Could you check a few things on this model? Use its own coordinates, in mm. A direction names the side the tool comes from. Round coordinates to 2 decimals unless told otherwise and drop trailing zeros. Order: outer loops, then holes, each group sorted by start corner. A loop starts at its lowest first (then second) coordinate and runs counter-clockwise, first axis right, second up. Notation, with made-up numbers: (37.25, -2) -> (45.25, -2) arc R9 cw to (45.25, 5) -> close; hole circle Ø2 at (72.5, -20). An arc over 180 degrees is marked (long way). One line per question, with ' | ' between items.
```python
from build123d import *

# Parameters (mm, degrees)
CYLINDER025_R          = 1
CYLINDER025_DEPTH      = 96
CYLINDER025_ROLL_ANGLE = -33
CYLINDER020_R          = 2
CYLINDER020_DEPTH      = 16
CYLINDER024_R          = 3
CYLINDER024_DEPTH      = 16
CYLINDER022_R          = 3
CYLINDER022_DEPTH      = 16
BOX021_W               = 26
BOX021_H               = 23
BOX021_DEPTH           = 13
CYLINDER011_R          = 1.9
CYLINDER011_DEPTH      = 12
CYLINDER012_R          = 1.9
CYLINDER012_DEPTH      = 12
CYLINDER013_R          = 1.9
CYLINDER013_DEPTH      = 12
CYLINDER014_R          = 1.9
CYLINDER014_DEPTH      = 12
BOX008_W               = 41
BOX008_H               = 20
BOX008_DEPTH           = 12
BOX019_W               = 10
BOX019_H               = 10
BOX019_DEPTH           = 10
BOX019_PLACEMENT_ANGLE = 8
BOX018_W               = 14
BOX018_H               = 10
BOX018_DEPTH           = 10
BOX018_PLACEMENT_ANGLE = 16
BOX017_W               = 65
BOX017_H               = 11
BOX017_DEPTH           = 10
BOX017_PLACEMENT_ANGLE = 15
BOX016_W               = 76
BOX016_H               = 10
BOX016_DEPTH           = 10
BOX015_W               = 49
BOX015_H               = 10
BOX015_DEPTH           = 10
BOX015_PLACEMENT_ANGLE = -19
BOX014_W               = 53
BOX014_H               = 10
BOX014_DEPTH           = 10
BOX014_PLACEMENT_ANGLE = -36
BOX013_W               = 13
BOX013_H               = 11
BOX013_DEPTH           = 10
BOX012_W               = 23
BOX012_H               = 17
BOX012_DEPTH           = 10
BOX011_W               = 41
BOX011_H               = 6
BOX011_DEPTH           = 10
CYLINDER016_R          = 43
CYLINDER016_DEPTH      = 10
CYLINDER015_R          = 13
CYLINDER015_DEPTH      = 10
BOX010_W               = 37
BOX010_H               = 8
BOX010_DEPTH           = 12
BOX009_W               = 184
BOX009_H               = 34
BOX009_DEPTH           = 6
CHAMFER_SIZE           = 6
CHAMFER001_SIZE        = 1
CUT025_PITCH_ANGLE     = 90
FILLET_R               = 3
FILLET001_R            = 3
CUT035_ROLL_ANGLE      = -45
BOX024_W               = 10
BOX024_H               = 10
BOX024_DEPTH           = 13
CHAMFER002_SIZE        = 3
CHAMFER003_SIZE        = 3


with BuildPart() as cylinder025:
    # Cylinder025 → Cylinder025 (new body)
    with BuildSketch(Plane.XY):
        Circle(CYLINDER025_R)
    extrude(amount=CYLINDER025_DEPTH)


with BuildPart() as cylinder025_1:
    # Cylinder025 roll: moved
    add(cylinder025.part.rotate(Axis((0, 0, 0), (1, 0, 0)), CYLINDER025_ROLL_ANGLE))


with BuildPart() as cylinder025_2:
    # Cylinder025 placement: moved
    add(cylinder025_1.part.moved(Location((-2.5, 14, 31))))


with BuildPart() as cylinder020:
    # Cylinder020 → Cylinder020 (new body)
    with BuildSketch(Plane.XY.offset(9)):
        Circle(CYLINDER020_R)
    extrude(amount=CYLINDER020_DEPTH)


with BuildPart() as cylinder024:
    # Cylinder024 → Cylinder024 (new body)
    with BuildSketch(Plane.XY.offset(23)):
        Circle(CYLINDER024_R)
    extrude(amount=CYLINDER024_DEPTH)


with BuildPart() as not_used_cylinder001:
    # Cylinder022 → Cylinder022 (new body)
    with BuildSketch(Plane(origin=(0, -50, 23), x_dir=(1, 0, 0), z_dir=(0, 0, 1))):
        Circle(CYLINDER022_R)
    extrude(amount=CYLINDER022_DEPTH)


with BuildPart() as cube021:
    # Box021 → Box021 (new body)
    with BuildSketch(Plane(origin=(161, 15, -3), x_dir=(1, 0, 0), z_dir=(0, 0, 1))):
        with Locations((13, 11.5)):
            Rectangle(BOX021_W, BOX021_H)
    extrude(amount=BOX021_DEPTH)


with BuildPart() as cylinder011:
    # Cylinder011 → Cylinder011 (new body)
    with BuildSketch(Plane(origin=(38, 19.5, -1), x_dir=(1, 0, 0), z_dir=(0, 0, 1))):
        Circle(CYLINDER011_R)
    extrude(amount=CYLINDER011_DEPTH)


with BuildPart() as cylinder012:
    # Cylinder012 → Cylinder012 (new body)
    with BuildSketch(Plane(origin=(38, 29, -1), x_dir=(1, 0, 0), z_dir=(0, 0, 1))):
        Circle(CYLINDER012_R)
    extrude(amount=CYLINDER012_DEPTH)


with BuildPart() as cylinder013:
    # Cylinder013 → Cylinder013 (new body)
    with BuildSketch(Plane(origin=(87, 29, -1), x_dir=(1, 0, 0), z_dir=(0, 0, 1))):
        Circle(CYLINDER013_R)
    extrude(amount=CYLINDER013_DEPTH)


with BuildPart() as cylinder014:
    # Cylinder014 → Cylinder014 (new body)
    with BuildSketch(Plane(origin=(87, 19.5, -1), x_dir=(1, 0, 0), z_dir=(0, 0, 1))):
        Circle(CYLINDER014_R)
    extrude(amount=CYLINDER014_DEPTH)


with BuildPart() as cube008:
    # Box008 → Box008 (new body)
    with BuildSketch(Plane(origin=(42, 14, -1), x_dir=(1, 0, 0), z_dir=(0, 0, 1))):
        with Locations((20.5, 10)):
            Rectangle(BOX008_W, BOX008_H)
    extrude(amount=BOX008_DEPTH)


with BuildPart() as cube019:
    # Box019 → Box019 (new body)
    with BuildSketch(Plane.XY):
        with Locations((5, 5)):
            Rectangle(BOX019_W, BOX019_H)
    extrude(amount=BOX019_DEPTH)


with BuildPart() as cube019_1:
    # Box019 placement: moved
    add(cube019.part.moved(Location((106, -7, 0))).rotate(Axis((106, -7, 0), (0, 0, 1)), BOX019_PLACEMENT_ANGLE))


with BuildPart() as cube018:
    # Box018 → Box018 (new body)
    with BuildSketch(Plane.XY):
        with Locations((7, 5)):
            Rectangle(BOX018_W, BOX018_H)
    extrude(amount=BOX018_DEPTH)


with BuildPart() as cube018_1:
    # Box018 placement: moved
    add(cube018.part.moved(Location((174, 10, 0))).rotate(Axis((174, 10, 0), (0, 0, 1)), BOX018_PLACEMENT_ANGLE))


with BuildPart() as cube017:
    # Box017 → Box017 (new body)
    with BuildSketch(Plane.XY):
        with Locations((32.5, 5.5)):
            Rectangle(BOX017_W, BOX017_H)
    extrude(amount=BOX017_DEPTH)


with BuildPart() as cube017_1:
    # Box017 placement: moved
    add(cube017.part.moved(Location((115, -7, 0))).rotate(Axis((115, -7, 0), (0, 0, 1)), BOX017_PLACEMENT_ANGLE))


with BuildPart() as cube016:
    # Box016 → Box016 (new body)
    with BuildSketch(Plane(origin=(46, -7, 0), x_dir=(1, 0, 0), z_dir=(0, 0, 1))):
        with Locations((38, 5)):
            Rectangle(BOX016_W, BOX016_H)
    extrude(amount=BOX016_DEPTH)


with BuildPart() as cube015:
    # Box015 → Box015 (new body)
    with BuildSketch(Plane.XY):
        with Locations((24.5, 5)):
            Rectangle(BOX015_W, BOX015_H)
    extrude(amount=BOX015_DEPTH)


with BuildPart() as cube015_1:
    # Box015 placement: moved
    add(cube015.part.moved(Location((16, 5, 0))).rotate(Axis((16, 5, 0), (0, 0, 1)), BOX015_PLACEMENT_ANGLE))


with BuildPart() as cube014:
    # Box014 → Box014 (new body)
    with BuildSketch(Plane.XY):
        with Locations((26.5, 5)):
            Rectangle(BOX014_W, BOX014_H)
    extrude(amount=BOX014_DEPTH)


with BuildPart() as cube014_1:
    # Box014 placement: moved
    add(cube014.part.moved(Location((-16, 28, 0))).rotate(Axis((-16, 28, 0), (0, 0, 1)), BOX014_PLACEMENT_ANGLE))


with BuildPart() as cube013:
    # Box013 → Box013 (new body)
    with BuildSketch(Plane(origin=(0, 8, 0), x_dir=(1, 0, 0), z_dir=(0, 0, 1))):
        with Locations((6.5, 5.5)):
            Rectangle(BOX013_W, BOX013_H)
    extrude(amount=BOX013_DEPTH)


with BuildPart() as cube012:
    # Box012 → Box012 (new body)
    with BuildSketch(Plane(origin=(161, 0, 0), x_dir=(1, 0, 0), z_dir=(0, 0, 1))):
        with Locations((11.5, 8.5)):
            Rectangle(BOX012_W, BOX012_H)
    extrude(amount=BOX012_DEPTH)


with BuildPart() as cube011:
    # Box011 → Box011 (new body)
    with BuildSketch(Plane(origin=(120, 0, 0), x_dir=(1, 0, 0), z_dir=(0, 0, 1))):
        with Locations((20.5, 3)):
            Rectangle(BOX011_W, BOX011_H)
    extrude(amount=BOX011_DEPTH)


with BuildPart() as cylinder016:
    # Cylinder016 → Cylinder016 (new body)
    with BuildSketch(Plane(origin=(132, 63, 0), x_dir=(1, 0, 0), z_dir=(0, 0, 1))):
        Circle(CYLINDER016_R)
    extrude(amount=CYLINDER016_DEPTH)


with BuildPart() as cylinder015:
    # Cylinder015 → Cylinder015 (new body)
    with BuildSketch(Plane(origin=(20, 37, 0), x_dir=(1, 0, 0), z_dir=(0, 0, 1))):
        Circle(CYLINDER015_R)
    extrude(amount=CYLINDER015_DEPTH)


with BuildPart() as cube010:
    # Box010 → Box010 (new body)
    with BuildSketch(Plane.XY):
        with Locations((18.5, 4)):
            Rectangle(BOX010_W, BOX010_H)
    extrude(amount=BOX010_DEPTH)


with BuildPart() as cut035:
    # Box009 → Box009 (new body)
    with BuildSketch(Plane.XY):
        with Locations((92, 17)):
            Rectangle(BOX009_W, BOX009_H)
    extrude(amount=BOX009_DEPTH)

    # Cut008: cut Cube010
    add(cube010.part, mode=Mode.SUBTRACT)

    # Cut009: cut Cylinder015
    add(cylinder015.part, mode=Mode.SUBTRACT)

    # Cut010: cut Cylinder016
    add(cylinder016.part, mode=Mode.SUBTRACT)

    # Cut011: cut Cube011
    add(cube011.part, mode=Mode.SUBTRACT)

    # Cut012: cut Cube012
    add(cube012.part, mode=Mode.SUBTRACT)

    # Cut013: cut Cube013
    add(cube013.part, mode=Mode.SUBTRACT)

    # Cut014: cut Cube014
    add(cube014_1.part, mode=Mode.SUBTRACT)

    # Cut015: cut Cube015
    add(cube015_1.part, mode=Mode.SUBTRACT)

    # Cut016: cut Cube016
    add(cube016.part, mode=Mode.SUBTRACT)

    # Cut017: cut Cube017
    add(cube017_1.part, mode=Mode.SUBTRACT)

    # Cut018: cut Cube018
    add(cube018_1.part, mode=Mode.SUBTRACT)

    # Cut019: cut Cube019
    add(cube019_1.part, mode=Mode.SUBTRACT)

    # Cut020: cut Cube008
    add(cube008.part, mode=Mode.SUBTRACT)

    # Cut021: cut Cylinder014
    add(cylinder014.part, mode=Mode.SUBTRACT)

    # Cut022: cut Cylinder013
    add(cylinder013.part, mode=Mode.SUBTRACT)

    # Cut023: cut Cylinder012
    add(cylinder012.part, mode=Mode.SUBTRACT)

    # Cut024: cut Cylinder011
    add(cylinder011.part, mode=Mode.SUBTRACT)

    # Chamfer
    chamfer_edges = [cut035.edges().sort_by_distance(p)[0] for p in [
        (7.350889, 34, 3),
    ]]
    chamfer(chamfer_edges, length=CHAMFER_SIZE)

    # Chamfer001
    chamfer001_edges = [cut035.edges().sort_by_distance(p)[0] for p in [
        (100.250984, 34, 3),
    ]]
    chamfer(chamfer001_edges, length=CHAMFER001_SIZE)

    # Cut025: cut Cube021
    add(cube021.part, mode=Mode.SUBTRACT)


with BuildPart() as cut035_1:
    # Cut025 pitch: moved
    add(cut035.part.rotate(Axis((0, 0, 0), (0, 1, 0)), CUT025_PITCH_ANGLE))


with BuildPart() as cut035_2:
    # Cut025 placement: moved
    add(cut035_1.part.moved(Location((-5.5, -24, 171))))

    # Fillet
    fillet_edges = [cut035_2.edges().sort_by_distance(p)[0] for p in [
        (-2.5, 7.250984, 10),
    ]]
    fillet(fillet_edges, radius=FILLET_R)

    # Fillet001
    fillet001_edges = [cut035_2.edges().sort_by_distance(p)[0] for p in [
        (-2.5, -7.286299, 10),
    ]]
    fillet(fillet001_edges, radius=FILLET001_R)

    # Cut035: cut Not used cylinder001
    add(not_used_cylinder001.part, mode=Mode.SUBTRACT)


with BuildPart() as cut035_3:
    # Cut035 roll: moved
    add(cut035_2.part.rotate(Axis((0, 0, 0), (1, 0, 0)), CUT035_ROLL_ANGLE))


with BuildPart() as cut035_4:
    # Cut035 placement: moved
    add(cut035_3.part.moved(Location((0, -8, 5))))


with BuildPart() as leg:
    # Box024 → Box024 (new body)
    with BuildSketch(Plane(origin=(-5.5, -5.5, 10), x_dir=(1, 0, 0), z_dir=(0, 0, 1))):
        with Locations((5, 5)):
            Rectangle(BOX024_W, BOX024_H)
    extrude(amount=BOX024_DEPTH)

    # Fusion006: union Cut035
    add(cut035_4.part)

    # Cut036: cut Cylinder024
    add(cylinder024.part, mode=Mode.SUBTRACT)

    # Cut037: cut Cylinder020
    add(cylinder020.part, mode=Mode.SUBTRACT)

    # Chamfer002
    chamfer002_edges = [leg.edges().sort_by_distance(p)[0] for p in [
        (4.5, 4.5, 16.5),
    ]]
    chamfer(chamfer002_edges, length=CHAMFER002_SIZE)

    # Chamfer003
    chamfer003_edges = [leg.edges().sort_by_distance(p)[0] for p in [
        (4.5, -5.5, 16.5),
    ]]
    chamfer(chamfer003_edges, length=CHAMFER003_SIZE)

    # Cut038: cut Cylinder025
    add(cylinder025_2.part, mode=Mode.SUBTRACT)


solid = leg.part
```
1. I want a section at C-C on z = 107. List the corners of the cut face in (x, y) for me, and give its area (3 significant figures).
From the geometry:
outline: (-5.5, 67.85) -> (0.5, 67.85) -> (0.5, 95.74) -> (-5.5, 95.74) -> close | area: 167 mm²
2. I'm going to push flat-ended pins straight in: pin 1 (2.5 mm diameter, centred on y = 82.86, z = 102.23, fed in from +X); pin 2 (3 mm diameter, centred on x = 0.5, y = 1.5, fed in from +Z); pin 3 (2 mm diameter, centred on x = -1, z = 17, fed in from +Y); pin 4 (2 mm diameter, centred on x = -3.5, z = 39, fed in from -Y). Where does each tip first touch, or does it pass through?
From the geometry:
pin 1: passes through | pin 2: stops at z = 32.95 | pin 3: stops at y = 6.17 | pin 4: stops at y = 5.91
3. I want a section at B-B on y = 72. List the corners of the cut face in (x, z) for me.
From the geometry:
outline: (-5.5, 99.14) -> (0.5, 99.14) -> (0.5, 109.03) -> (-5.5, 109.03) -> close
4. If we mould it in two halves opening along X, with no side actions, what happens to faces 1 (the face through (3, 3, 16)), 2 (the face through (0, -2, 16)), 3 (the face through (-2.458, 113.992, 116.694))? For each: pulls with the +X half, pulls with the -X half, needs draft (parallel to the pull), parting line crosses it, or undercut.
From the geometry:
face 1: pulls with the +X half | face 2: undercut | face 3: needs draft
5. I want a section at A-A on y = 0. List the corners of the cut face in (x, z) for me.
From the geometry:
outline: (-5.5, 10) -> (-2, 10) -> (-2, 23) -> (-3, 23) -> (-3, 27.76) -> (-5.5, 27.76) -> close; (2, 10) -> (4.5, 10) -> (4.5, 23) -> (2, 23) -> close
6. On a 3-axis mill with a long thin cutter (end or side, diameter ignored), from which of +Z, -Z, +X, -X, +Y, -Y can I reach the whole of each face in a straight line? I mean faces 4 (the face through (1, 4.5, 14)), 5 (the face through (-2.542, 48.464, 69.463)). Say none if no direction works.
From the geometry:
face 4: -Z, +X, +Y | face 5: +X, -X
7. I need wall thicknesses on probe 1 along Y at (x, z) = (-2, 100.5); probe 2 along Z at (x, y) = (-0.25, 58); probe 3 along X at (y, z) = (65, 105.5). Which ranges of each line are inside material? Lowest first, please.
From the geometry:
probe 1: y = 57.8 to 58.1, 60.17 to 73.36, 78.93 to 82.07, 83.65 to 95.13 | probe 2: z = 56.86 to 63.45, 85.14 to 100.7 | probe 3: x = -5.5 to 0.5
